Autodesk Inventor part; units mm, degrees
ref_plane "YZ Plane" through (0, 0, 0) normal (1, 0, 0) x (0, 1, 0)
ref_plane "XZ Plane" through (0, 0, 0) normal (0, 1, 0) x (-1, 0, 0)
ref_plane "XY Plane" through (0, 0, 0) normal (0, 0, 1) x (1, 0, 0)
sketch "Boceto1" plane through (0, 0, 0) normal (0, 0, 1) x (1, 0, 0)
  line L0 (0, 0) -> (-20, 0)
  line L1 (-20, 0) -> (0, 0)
  line L2 (-20, 0) -> (0, 0)
  line L3 (-65, -10) -> (65, -10)
  line L4 (65, -10) -> (65, 10)
  line L5 (65, 10) -> (-65, 10)
  line L6 (-65, 10) -> (-65, -10)
  circle A0 centre (-10, 0) radius 25
  point P0 (-20, -35)
  point P1 (12.9129, 10)
  point P2 (-32.9129, 10)
  point P3 (-32.9129, -10)
  point P4 (12.9129, -10)
  dimension "d4" = 20
  dimension "d6" = 130
  dimension "d7" = 20
  dimension "d8" = 50
extrude "Extrusión1" add sketch "Boceto1" along normal blind 5.5
sketch "Boceto2" plane through (0, 0, 5.5) normal (0, 0, 1) x (1, 0, 0)
  line L0 (65, -10) -> (65, 10)
  line L1 (65, 0) -> (90, 0)
  line L2 (65, 0) -> (85, 0)
  line L3 (85, 0) -> (90, 0)
  circle A0 centre (87.5, 0) radius 1.5
  line L4 (65, 0) -> (95, 0)
  line L5 (95, 0) -> (95, -10)
  line L6 (12.9129, -10) -> (65, -10)
  line L7 (95, -10) -> (65, -10)
  line L8 (65, -10) -> (65, 10)
  line L9 (95, 10) -> (65, 10)
  line L10 (95, 0) -> (95, 10)
  arc A1 (95, -2.0554) -> (95, 0) centre (85.9536, -1.0277) ccw
  arc A2 (95, 0) -> (95, 2.0554) centre (85.9536, 1.0277) ccw
  arc A3 (85, -10) -> (85, 10) centre (85, 0) ccw
  point P0 (0, 0)
  point P1 (87.5, -10)
  point P2 (87.5, 10)
  point P3 (95, 2.0554)
  point P4 (87.5, 10)
  point P5 (95, -2.0554)
  dimension "d11" = 25
  dimension "d12" = 20
  dimension "d13" = 3
  dimension "d14" = 30
extrude "Extrusión2" add sketch "Boceto2" against normal blind 5.5 contours L0 L1 A0 L4 A3 L7 | L0 L9 A3 L4 L1 A0
sketch "Boceto4" plane through (0, 0, 5.5) normal (0, 0, 1) x (1, 0, 0)
  line L0 (-65, 10) -> (-65, -10)
  line L1 (-65, 0) -> (-95, 0)
  line L2 (-95, 0) -> (-95, 10)
  line L3 (-95, 10) -> (-65, 10)
  line L4 (-65, -10) -> (-95, -10)
  line L5 (-95, -10) -> (-95, 0)
  line L6 (-65, 0) -> (-85, 0)
  arc A0 (-85, 10) -> (-85, -10) centre (-85, 0) ccw
  point P0 (0, 0)
  dimension "d17" = 30
  dimension "d18" = 20
extrude "Extrusión3" add sketch "Boceto4" against normal blind 5.5 contours L0 L1 A0 L3 | L0 L4 A0 L1
properties part number "lamina"
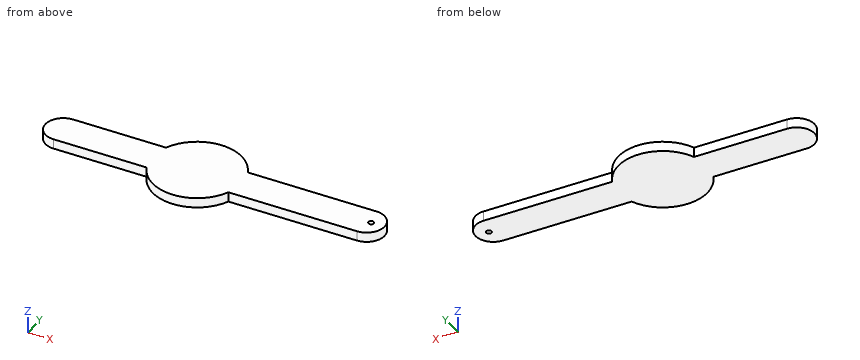
Work out the finished part from the listing and answer in its coordinate system (mm). Give positions to 0.01 mm unless a question says otherwise; leave off trailing zeros. Loops run counter-clockwise (first coordinate to the right, second up) from the corner with the lowest first, then second, coordinate; pieces in that order, holes last. Notation, with made-up numbers: (72.5, 57.25) -> (120.5, 57.25) arc R21 cw to (120.5, 73.25) -> close; hole circle Ø9 at (-28.75, 81). An arc over 180 degrees is marked (long way). Put each result on its own line as item: value. Start each with the question number.
Item 1: Find the intervals of material crossed by L1, parallel to X at y = 0, z = 3.75; L2, parallel to Y at x = 59, z = 5.1; L3, parallel to Y at x = 87.5, z = 1.3, in increasing order. Write a range as [from, to].
Item 2: Each of these flat-tipped pins is pushed along its axis until it touches: P1, Ø3, axis at x = 34.5, z = 2.5, coming from the -Y side; P2, Ø5, axis at x = 87.5, y = 0, coming from the +Z side; P3, Ø3, axis at x = -58, z = 4, coming from the +Y side; P4, Ø12, axis at x = 20.5, y = -19, coming from the +Z side. Where does it stop, or does it pass through?
Item 3: The part is cut by section B-B (x = 63). Give the vertices of the cut face in (y, z).
Item 4: The part is cut by section C-C (y = 16). Give the vertices of the cut face in (x, z), then the cut area to 3 significant figures.
Item 5: The part is cut by section A-A (z = 3.55). Give the vertices of the cut face in (x, y), then the cut area to 3 significant figures.
Answers below:
1. L1: [-95, 86], [89, 95]
1. L2: [-10, 10]
1. L3: [-9.68, -1.5], [1.5, 9.68]
2. P1: y = -10
2. P2: z = 5.5
2. P3: y = 10
2. P4: through
3. outline: (-10, 0) -> (10, 0) -> (10, 5.5) -> (-10, 5.5) -> close
4. outline: (-29.21, 0) -> (9.21, 0) -> (9.21, 5.5) -> (-29.21, 5.5) -> close
4. area: 211 mm2
5. outline: (-85, -10) -> (-32.91, -10) arc R25 ccw to (12.91, -10) -> (85, -10) arc R10 ccw to (85, 10) -> (12.91, 10) arc R25 ccw to (-32.91, 10) -> (-85, 10) arc R10 ccw to start; hole circle Ø3 at (87.5, 0)
5. area: 4,700 mm2
